Read the model definition and answer for the solid it produces. Units are mm, in the model's axes. Face numbers are marked on the shaded views. Give positions to 0.01 mm unless a question says otherwise; leave off trailing zeros. Order: outer loops, then holes, each group sorted by start corner. A loop starts at its lowest first (then second) coordinate and runs counter-clockwise, first axis right, second up. Notation, with made-up numbers: M 29,65.25 L 44,65.25 A12 cw 44,78.25 Z; hole C 13,74.25 d2. An arc over 180 degrees is marked long. One line per item, written item: value. Start each with the question number.
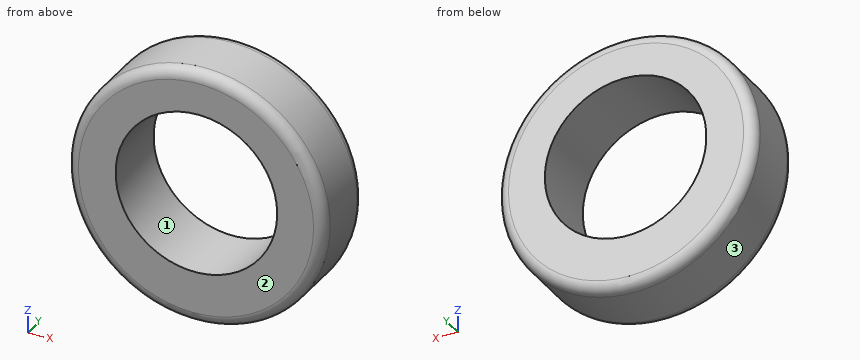
from build123d import *

# Parameters (mm, degrees)
F0_R     = 44.45
F1_DEPTH = 12.7
F2_R     = 3.81
F3_R     = 27.94
F4_DEPTH = 25.401


with BuildPart() as f1:
    # F0 (on Front) → F1 (new body, symmetric)
    with BuildSketch(Plane.XZ):
        with Locations((30.440104, -5.716477)):
            Circle(F0_R)
    extrude(amount=F1_DEPTH, both=True)

    # F2
    f2_edges = [f1.edges().sort_by_distance(p)[0] for p in [
        (-14.009896, -12.7, -5.716477),
        (-14.009896, 12.7, -5.716477),
    ]]
    fillet(f2_edges, radius=F2_R)

    # F3 (on face) → F4 (cut, through all)
    with BuildSketch(Plane.XZ.offset(12.7)):
        with Locations((30.583977, -3.976314)):
            Circle(F3_R)
    extrude(amount=-F4_DEPTH, mode=Mode.SUBTRACT)


solid = f1.part
Q1. Find section B-B, the plane y = 6.75. Give the vertices of the cut face in (x, z).
Q2. Determine the mould class of the marked faces 1, 2 and 3 for opening direction X: released by +X, released by -X, zero draft, split by the parting line, or undercut.
Q3. Each of these flat-tipped pins is pushed along its axis until it touches: pin 1 (8 mm diameter, centred on y = 5, z = 16.5, fed in from +X); pin 2 (10 mm diameter, centred on y = 1, z = -36, fed in from -X); pin 3 (1.5 mm diameter, centred on x = 62, y = 7, fed in from -Z). Where does it stop, or does it pass through?
Q4. Consider probe 1 along Z at (x, y) = (9.5, -2.75); probe 2 along Z at (x, y) = (28, 6.75); probe 3 along X at (y, z) = (2, -8.5). Determine where each line is inside the solid, lowest interval first.
Q5. Find section A-A, the plane y = -10. Give the vertices of the cut face in (x, z).
Evaluation:
1. outline: C 30.44,-5.72 d88.9; hole C 30.58,-3.98 d55.88
2. face 1: undercut
2. face 2: zero draft
2. face 3: split by the parting line
3. pin 1: x = 70.99
3. pin 2: x = -6.12
3. pin 3: z = -37.76
4. probe 1: -44.93 to -22.31, 14.36 to 33.49
4. probe 2: -50.1 to -31.8, 23.84 to 38.67
4. probe 3: -13.92 to 3.01, 58.16 to 74.8
5. outline: C 30.44,-5.72 d88.57; hole C 30.58,-3.98 d55.88
